Autodesk Inventor part; units mm, degrees
ref_plane "YZ Plane" through (0, 0, 0) normal (1, 0, 0) x (0, 1, 0)
ref_plane "XZ Plane" through (0, 0, 0) normal (0, 1, 0) x (-1, 0, 0)
ref_plane "XY Plane" through (0, 0, 0) normal (0, 0, 1) x (1, 0, 0)
sketch "Sketch1" plane through (0, 0, 0) normal (0, 1, 0) x (-1, 0, 0)
  line L0 (0, 0) -> (50.8, 0)
  line L1 (50.8, 0) -> (50.8, -25.4)
  line L2 (50.8, -25.4) -> (0, -25.4)
  line L3 (0, -25.4) -> (0, 0)
  dimension "d0" = 50.8
  dimension "d1" = 25.4
  dimension "d2" = 50.8
  dimension "d3" = 90
extrude "Extrusion1" add sketch "Sketch1" along normal blind 12.7
sketch "Sketch2" plane through (0, 0, -25.4) normal (0, 0, -1) x (-1, 0, 0)
  line L0 (0, 12.7) -> (50.8, 12.7)
  line L1 (50.8, 12.7) -> (12.7, 12.7)
  line L2 (12.7, 12.7) -> (12.7, -76.2)
  line L3 (12.7, 12.7) -> (88.9, 12.7)
  line L4 (88.9, 12.7) -> (88.9, -38.1)
  line L5 (88.9, -38.1) -> (12.7, -38.1)
  line L6 (12.7, -38.1) -> (12.7, 12.7)
  point P0 (0, 0)
  point P1 (12.7, -38.1)
  dimension "d11" = 76.2
  dimension "d12" = 50.8
extrude "Extrusion2" add sketch "Sketch2" along normal blind 12.7
move or copy body "Move Body1" bodies to move or copy 1 copy no rotation origin (0, 0, 0) rotation axis (0, 1, 0) rotation angle -90 translate (-76.2, 0, 25.4)
properties part number "wobble goal arm"
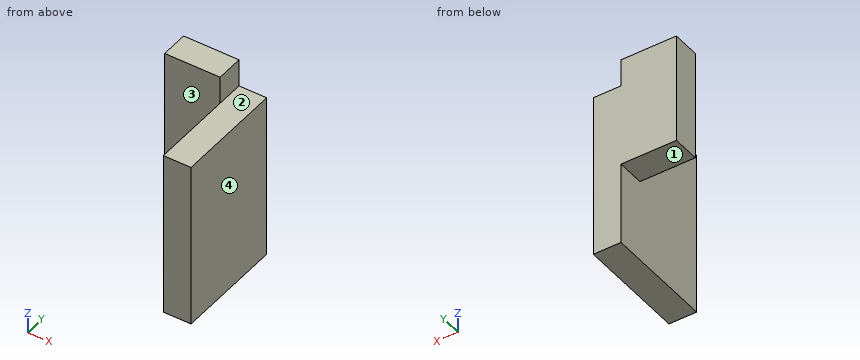
Can you work these out from the model? Positions are in its coordinate system, mm. Face numbers are marked on the shaded views. A direction names the side the tool comes from. Round coordinates to 2 decimals unless told otherwise and drop trailing zeros. Loops run counter-clockwise (first coordinate to the right, second up) from the corner with the lowest first, then second, coordinate; pieces in that order, holes last. Notation, with made-up numbers: (85, 2) - (97, 2) arc R21 cw to (97, 31) - close; hole circle Ø1 at (70, -4). An arc over 180 degrees is marked (long way). Use CSV: the item, a comma, the result in double quotes. Start each with the question number.
1) For pin 1 Ø12 at (y, z) = (-15.5, 2.5) entering from -X; pin 2 Ø6.5 at (y, z) = (9.5, 18.5) entering from +X; pin 3 Ø20.5 at (x, z) = (-69.5, 6) entering from -Y, each with a flat end and sliding along its axis, tell me the tip position at first contact or that it passes through.
2) If we section it at B-B on z = -23.5: Write out the boundary of the cut face in (x, y), plus the area to 3 significant figures.
3) If we section it at D-D on z = -44.5: Write out the boundary of the cut face in (x, y), plus the area to 3 significant figures.
4) If we section it at C-C on x = -41.5: Write out the boundary of the cut face in (y, z).
5) If we section it at A-A on y = 6.5: Write out the boundary of the cut face in (x, z), plus the area to 3 significant figures.
6) Please list where these lines run through material, in increasing order: probe 1 along X at (y, z) = (-18, -27.5); probe 2 along Z at (x, y) = (-51.5, 7.5); probe 3 along Y at (x, z) = (-52, 9). Write a range as [from, to].
7) For the marked faces 1, 2, 3 and 4, which set-ups out of +Z, -Z, +X, -X, +Y, -Y let a thin tool reach every point of the face, with its end or its side?
Geometry results:
1,pin 1,"stops at x = -50.8"
1,pin 2,"stops at x = -50.8"
1,pin 3,"stops at y = 0"
2,outline,"(-76.2, 0) - (-50.8, 0) - (-50.8, -38.1) - (-38.1, -38.1) - (-38.1, 12.7) - (-76.2, 12.7) - close"
2,area,"968 mm2"
3,outline,"(-50.8, -38.1) - (-38.1, -38.1) - (-38.1, 12.7) - (-50.8, 12.7) - close"
3,area,"645 mm2"
4,outline,"(-38.1, -63.5) - (12.7, -63.5) - (12.7, 12.7) - (-38.1, 12.7) - close"
5,outline,"(-76.2, -25.4) - (-50.8, -25.4) - (-50.8, -63.5) - (-38.1, -63.5) - (-38.1, 12.7) - (-50.8, 12.7) - (-50.8, 25.4) - (-76.2, 25.4) - close"
5,area,"2,260 mm2"
6,probe 1,"x = [-50.8, -38.1]"
6,probe 2,"z = [-25.4, 25.4]"
6,probe 3,"y = [0, 12.7]"
7,face 1,"-Z, -X, +Y, -Y"
7,face 2,"+Z, +X, +Y, -Y"
7,face 3,"+Z, -Z, -X, -Y"
7,face 4,"+Z, -Z, +X, +Y, -Y"
